Geometry: final body of the model. Coordinates: model frame, mm. Round coordinates to 2 decimals unless told otherwise and drop trailing zeros. Write each loop counter-clockwise with the first axis right and the second up, starting at its lowest first coordinate (ties: lowest second). Pieces come first, ordered by that corner, then holes. Notation, with made-up numbers: (31.5, 88.25) - (72.5, 88.25) arc R11 cw to (72.5, 107.25) - close; hole circle Ø6 at (-35, -22). An arc over 180 degrees is marked (long way). Write each question's results on one line, items separated by ' | '.
from build123d import *

# Parameters (mm, degrees)
SKETCH1_W           = 65
SKETCH1_H           = 90
BOSS_EXTRUDE1_DEPTH = 3
SKETCH3_R           = 1.5
CUT_EXTRUDE2_DEPTH  = 3
SKETCH4_R           = 1.5
CUT_EXTRUDE3_DEPTH  = 4
SKETCH5_W           = 3
SKETCH5_H           = 32
CUT_EXTRUDE4_DEPTH  = 4
SKETCH6_W           = 3
SKETCH6_H           = 22
CUT_EXTRUDE5_DEPTH  = 4
SKETCH7_W           = 3
SKETCH7_H           = 30.5
SKETCH7_W_2         = 14
SKETCH7_H_2         = 7
SKETCH7_W_3         = 16
SKETCH7_H_3         = 8
CUT_EXTRUDE6_DEPTH  = 4
SKETCH8_W           = 12
SKETCH8_H           = 18.5
CUT_EXTRUDE7_DEPTH  = 4


with BuildPart() as part:
    # Sketch1 → Boss-Extrude1 (new body)
    with BuildSketch(Plane.XY):
        Rectangle(SKETCH1_W, SKETCH1_H)
    extrude(amount=-BOSS_EXTRUDE1_DEPTH)

    # Sketch3 → Cut-Extrude2 (cut)
    with BuildSketch(Plane.XY):
        with Locations((-8.98, 30.5)):
            Circle(SKETCH3_R)
        with Locations((-3.9, 2.56)):
            Circle(SKETCH3_R)
        with Locations((21.5, 2.56)):
            Circle(SKETCH3_R)
    extrude(amount=-CUT_EXTRUDE2_DEPTH, mode=Mode.SUBTRACT)

    # Sketch4 → Cut-Extrude3 (cut, through all)
    with BuildSketch(Plane.XY):
        with Locations((-15.25, -42.25)):
            Circle(SKETCH4_R)
        with Locations((-15.25, -11.75)):
            Circle(SKETCH4_R)
        with Locations((15.25, -42.25)):
            Circle(SKETCH4_R)
        with Locations((15.25, -11.75)):
            Circle(SKETCH4_R)
    extrude(amount=-CUT_EXTRUDE3_DEPTH, mode=Mode.SUBTRACT)

    # Sketch5 → Cut-Extrude4 (cut, through all)
    with BuildSketch(Plane.XY):
        with Locations((28, -19)):
            Rectangle(SKETCH5_W, SKETCH5_H)
        with Locations((28, 19)):
            Rectangle(SKETCH5_W, SKETCH5_H)
    extrude(amount=-CUT_EXTRUDE4_DEPTH, mode=Mode.SUBTRACT)

    # Sketch6 → Cut-Extrude5 (cut, through all)
    with BuildSketch(Plane.XY):
        with Locations((-28, -4)):
            Rectangle(SKETCH6_W, SKETCH6_H)
        with Locations((-28, 24)):
            Rectangle(SKETCH6_W, SKETCH6_H)
    extrude(amount=-CUT_EXTRUDE5_DEPTH, mode=Mode.SUBTRACT)

    # Sketch7 → Cut-Extrude6 (cut, through all)
    with BuildSketch(Plane.XY):
        with Locations((16.5, -27)):
            Rectangle(SKETCH7_W, SKETCH7_H)
        with Locations((-5.25, -12.75)):
            Rectangle(SKETCH7_W_2, SKETCH7_H_2)
        with Locations((4.25, -41)):
            Rectangle(SKETCH7_W_3, SKETCH7_H_3)
    extrude(amount=-CUT_EXTRUDE6_DEPTH, mode=Mode.SUBTRACT)

    # Sketch8 → Cut-Extrude7 (cut, through all)
    with BuildSketch(Plane.XY):
        with Locations((-26.5, -35.75)):
            Rectangle(SKETCH8_W, SKETCH8_H)
    extrude(amount=-CUT_EXTRUDE7_DEPTH, mode=Mode.SUBTRACT)


solid = part.part
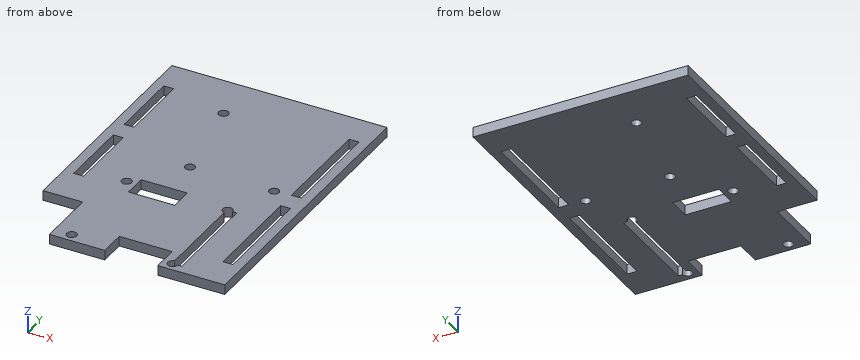
Q1. Section query B-B, the plane x = -15.25. Return loops of the section in (y, z).
Answer block:
outline: (-45, -3) - (-43.75, -3) - (-43.75, 0) - (-45, 0) - close; (-40.75, -3) - (-13.25, -3) - (-13.25, 0) - (-40.75, 0) - close; (-10.25, -3) - (45, -3) - (45, 0) - (-10.25, 0) - close
Q2. Ray query, line 1 along X through (y, z) = (-38, -0.45); line 2 along Y through (x, z) = (-15.25, -0.8); line 3 along Y through (x, z) = (28, -0.9). Return the intervals inside material, ascending.
Answer block:
line 1: -20.5 to -3.75, 12.25 to 15, 18 to 32.5 | line 2: -45 to -43.75, -40.75 to -13.25, -10.25 to 45 | line 3: -45 to -35, -3 to 3, 35 to 45
Q3. Section query A-A, the plane y = -38. Return loops of the section in (x, z), plus the area to 3 significant figures.
Answer block:
outline: (-20.5, -3) - (-3.75, -3) - (-3.75, 0) - (-20.5, 0) - close; (12.25, -3) - (15, -3) - (15, 0) - (12.25, 0) - close; (18, -3) - (32.5, -3) - (32.5, 0) - (18, 0) - close | area: 102 mm2
Q4. Section query C-C, the plane y = 30.5. Return loops of the section in (x, z), plus the area to 3 significant figures.
Answer block:
outline: (-32.5, -3) - (-29.5, -3) - (-29.5, 0) - (-32.5, 0) - close; (-26.5, -3) - (-10.48, -3) - (-10.48, 0) - (-26.5, 0) - close; (-7.48, -3) - (26.5, -3) - (26.5, 0) - (-7.48, 0) - close; (29.5, -3) - (32.5, -3) - (32.5, 0) - (29.5, 0) - close | area: 168 mm2
Q5. Section query D-D, the plane z = -2.3. Give the number of separate pieces and of enclosed holes in the cut face, plus the area to 3 significant figures.
Answer block:
separate pieces: 1 | enclosed holes: 11 | area: 4,940 mm2
Q6. Pin query (flat end, axial travel): pin 1 (3 mm diameter, centred on x = 2, y = 13, fed in from +Z); pin 2 (1.5 mm diameter, centred on y = -40, z = -1, fed in from -X); pin 3 (0.9 mm diameter, centred on x = -28, z = -1, fed in from -Y). Return the tip coordinate at first contact, or that it passes through.
Answer block:
pin 1: z = 0 | pin 2: x = -20.5 | pin 3: y = -26.5
